Part model, mm, in its own coordinate system. A direction names the side the tool comes from. Round coordinates to 2 decimals unless told otherwise and drop trailing zeros. Loops run counter-clockwise (first coordinate to the right, second up) from the corner with the lowest first, then second, coordinate; pieces in that order, holes last. Notation, with made-up numbers: M 83,63 L 114,63 A20 cw 114,87 Z; hole C -37,-18 d9. An arc over 180 degrees is marked long. Write each question's results on one line, items separated by ' | '.
Autodesk Inventor part; units mm, degrees
ref_plane "YZ Plane" through (0, 0, 0) normal (1, 0, 0) x (0, 1, 0)
ref_plane "XZ Plane" through (0, 0, 0) normal (0, 1, 0) x (-1, 0, 0)
ref_plane "XY Plane" through (0, 0, 0) normal (0, 0, 1) x (1, 0, 0)
sketch "Sketch1" plane through (0, 0, 0) normal (0, 1, 0) x (-1, 0, 0)
  arc A0 (-9.5, 10.9545) -> (9.5, 10.9545) centre (0, 0) ccw
  line L0 (-9.5, 10.9545) -> (-9.5, 20)
  line L1 (-9.5, 20) -> (9.5, 20)
  line L2 (9.5, 20) -> (9.5, 10.9545)
  line L3 (13.5, 12.6491) -> (13.5, 24)
  line L4 (13.5, 24) -> (-13.5, 24)
  line L5 (-13.5, 24) -> (-13.5, 12.6491)
  arc A1 (-13.5, 12.6491) -> (13.5, 12.6491) centre (0, 0) ccw
  point P0 (0, -20)
  point P1 (-9.5, 15)
  dimension "d0" = 0
  dimension "d1" = 29
  dimension "d6" = 20
  dimension "d7" = 19
  dimension "d8" = 4
extrude "Extrusion1" add sketch "Sketch1" along normal blind 18
sketch "Sketch2" plane through (0, 18, 0) normal (0, 1, 0) x (1, 0, 0)
  arc A0 (13.5, -12.6491) -> (-13.5, -12.6491) centre (0, 0) ccw
  line L0 (-13.5, -12.6491) -> (-13.5, -24)
  line L1 (-13.5, -24) -> (13.5, -24)
  line L2 (13.5, -24) -> (13.5, -12.6491)
  line L3 (-13.5, -12.6491) -> (-13.5, -24)
extrude "Extrusion2" add sketch "Sketch2" along normal blind 5
sketch "Sketch3" plane through (-13.5, 0, 24) normal (0, 0, 1) x (1, 0, 0)
  circle A0 centre (13.5, 0) radius 3.5
  dimension "d13" = 7
extrude "Extrusion3" cut sketch "Sketch3" against normal blind 5
sketch "Sketch4" plane through (0, 0, 0) normal (0, -1, 0) x (1, 0, 0)
  line L0 (0, 0) -> (-21, 0)
  line L1 (-21, -31.8183) -> (-51, -31.8183)
  line L2 (-51, -31.8183) -> (-51, 28.1817)
  line L3 (-51, 28.1817) -> (-21, 28.1817)
  line L4 (-21, 28.1817) -> (-21, -31.8183)
  line L5 (-13.5, 24) -> (13.5, 24)
  line L6 (-21, 28.1817) -> (-13.5, 24)
  line L7 (-21, -31.8183) -> (8.5554, -16.4029)
  arc A0 (-13.5, 12.6491) -> (13.5, 12.6491) centre (0, 0) ccw
  arc A1 (-13.5, 12.6491) -> (8.5554, -16.4029) centre (0, 0) ccw
  line L8 (-13.5, 12.6491) -> (-13.5, 24)
  line L9 (-13.5, 24) -> (-13.5, 12.6491)
  dimension "d19" = 21
  dimension "d20" = 30
  dimension "d21" = 60
extrude "Extrusion4" add sketch "Sketch4" against normal blind 23
sketch "Sketch6" plane through (-21, 0, -31.8183) normal (0, 0, -1) x (-1, 0, 0)
  line L0 (0, 0) -> (-29.5554, 0)
  line L1 (0, 0) -> (30.3611, 0)
  line L2 (30.3611, 0) -> (30.3611, 9.5813)
  line L3 (30.3611, 9.5813) -> (0, 9.5813)
  line L4 (0, 9.5813) -> (0, 0)
  point P0 (-21, 0)
  dimension "d26" = 9.5813
extrude "Extrusion5" cut sketch "Sketch6" against normal through all
properties part number "pitch_motor_standoff_v1"
Item 1: Which spindle directions (+Z, -Z, +X, -X, +Y, -Y) get a long thin tool onto all of the face, cutting with end or side? Do faces 4 (the flat face through (-21, 5, -2)), 5 (the flat face through (0, 11, 24)), 6 (the cylindrical face through (0.1, 3.5, 22)), 7 (the flat face through (9.5, 9, 15)), 8 (the flat face through (-14, 0, -8)). Say none if no direction does.
Filled sheet:
face 4: +Z, -Z, -X, -Y | face 5: +Z, +X, +Y, -Y | face 6: +Z, -Y | face 7: -Y | face 8: +Z, -Z, +X, -X, -Y
Item 2: Wall check: L1, parallel to X at y = 11, z = 0; L2, parallel to X at y = 8.5, z = 0; L3, parallel to Y at x = -41.5, z = -24. Give the ranges that are in metal, low to high.
Filled sheet:
L1: -51 to -14.5, 14.5 to 18.5 | L2: -21 to -14.5, 14.5 to 18.5 | L3: 9.58 to 23
Item 3: Band-saw the part on D-D on y = 19. Give the cut face in (x, z).
Filled sheet:
outline: M -51,-31.82 L -21,-31.82 L 8.56,-16.4 A18.5 ccw 13.5,12.65 L 13.5,24 L -13.5,24 L -21,28.18 L -51,28.18 Z
Item 4: Band-saw the part on C-C on x = 0. Give the cut face in (y, z), and give its area (3 significant figures).
Filled sheet:
outline: M 0,-20.87 L 23,-20.87 L 23,24 L 3.5,24 L 3.5,20 L 18,20 L 18,-14.5 L 0,-14.5 Z | area: 397 mm^2
Item 5: Band-saw the part on A-A on y = 11. Give the cut face in (x, z).
Filled sheet:
outline: M -51,-31.82 L -21,-31.82 L 8.56,-16.4 A18.5 ccw 13.5,12.65 L 13.5,24 L -13.5,24 L -21,28.18 L -51,28.18 Z; hole M -9.5,10.95 A14.5 ccw long 9.5,10.95 L 9.5,20 L -9.5,20 Z
Item 6: Drop flat-ended pins along their axis: P1, Ø9, axis at x = -3.5, y = 10, coming from the -Z side; P2, Ø3.5, axis at y = 7.5, z = 19.5, coming from the +X side; P3, Ø3, axis at y = 6, z = -20, coming from the +X side. Give the stop position or say it passes through.
Filled sheet:
P1: z = -25.04 | P2: x = 13.5 | P3: x = 4.53
Item 7: Two-plate mould, pull along Z, no slides. Class faces 1 (the cylindrical face through (-0.49, 8.87, -14.49)), 2 (the flat face through (-36, 16, -31.818)), 3 (the flat face through (-24, 23, -2)): +Z half, -Z half, draft (parallel to the pull), parting line (faces both ways), or undercut.
Filled sheet:
face 1: undercut | face 2: -Z half | face 3: draft
Item 8: Band-saw the part on B-B on z = 0. Give the cut face in (x, y).
Filled sheet:
outline: M -51,9.58 L -21,9.58 L -21,0 L -14.5,0 L -14.5,18 L 14.5,18 L 14.5,0 L 18.5,0 L 18.5,23 L -51,23 Z
